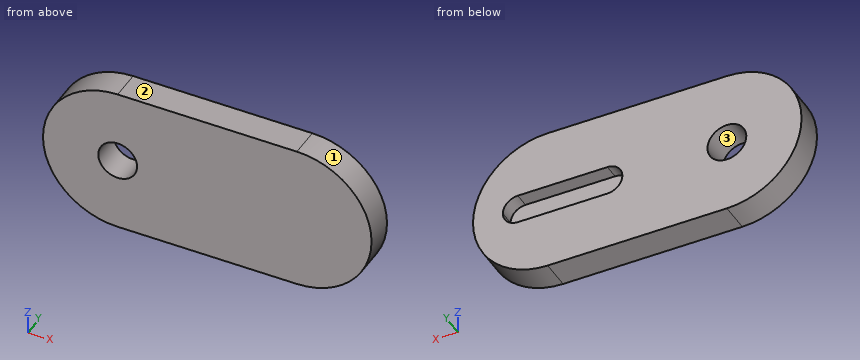
```python
from build123d import *

# Parameters (mm, degrees)
BOSS_EXTRUDE1_DEPTH = 2.54
SKETCH2_R           = 1.651
CUT_EXTRUDE1_DEPTH  = 2.54
SKETCH3_W           = 10.16
SKETCH3_H           = 2.54
CUT_EXTRUDE2_DEPTH  = 1.27
FILLET1_R           = 1.27


with BuildPart() as part:
    # Sketch1 → Boss-Extrude1 (new body)
    with BuildSketch(Plane(origin=(0, 0, 0), x_dir=(1, 0, 0), z_dir=(0, 1, 0))):
        with BuildLine():
            Line((0, 6.35), (15.24, 6.35))
            ThreePointArc((15.24, 6.35), (21.59, 0), (15.24, -6.35))
            Line((15.24, -6.35), (0, -6.35))
            ThreePointArc((0, -6.35), (-6.35, 0), (0, 6.35))
        make_face()
    extrude(amount=BOSS_EXTRUDE1_DEPTH)

    # Sketch2 → Cut-Extrude1 (cut)
    with BuildSketch(Plane(origin=(0, 2.54, 0), x_dir=(1, 0, 0), z_dir=(0, 1, 0))):
        with Locations(Location((0, 0, 0), (0, 0, 270))):
            Circle(SKETCH2_R)
    extrude(amount=-CUT_EXTRUDE1_DEPTH, mode=Mode.SUBTRACT)

    # Sketch3 → Cut-Extrude2 (cut)
    with BuildSketch(Plane(origin=(0, 2.54, 0), x_dir=(1, 0, 0), z_dir=(0, 1, 0))):
        with Locations((13.97, 0)):
            Rectangle(SKETCH3_W, SKETCH3_H)
    extrude(amount=-CUT_EXTRUDE2_DEPTH, mode=Mode.SUBTRACT)

    # Fillet1
    fillet1_edges = [part.edges().sort_by_distance(p)[0] for p in [
        (19.05, 1.905, 1.27),
        (19.05, 1.905, -1.27),
        (8.89, 1.905, 1.27),
        (8.89, 1.905, -1.27),
    ]]
    fillet(fillet1_edges, radius=FILLET1_R - 0.0001)  # a hair under: the kernel refuses the full size


solid = part.part
```
Check sheet for the modelled part. Datum: model origin and axes. Units: mm. Face numbers are marked on the shaded views. Give positions to 0.01 mm unless a question says otherwise; leave off trailing zeros. Loops run counter-clockwise (first coordinate to the right, second up) from the corner with the lowest first, then second, coordinate; pieces in that order, holes last. Notation, with made-up numbers: (-22.75, 9.5) - (34.25, 9.5) arc R16 cw to (34.25, 17.5) - close; hole circle Ø9 at (77, -38). An arc over 180 degrees is marked (long way). One line per question, with ' | ' between items. Start each with the question number.
1. Cross-section at B-B, the plane y = 1.55. Give the number of separate pieces and of enclosed holes in the cut face, plus the area to 3 significant figures.
2. Draft check along Z on the marked faces 1, 2 and 3. Enter one of: released by +Z, released by -Z, zero draft, split by the parting line, or undercut.
3. Material ranges on line 1 along X through (y, z) = (1.85, 0); line 2 along X through (y, z) = (1.2, 0); line 3 along Z through (x, y) = (11.75, 2.25), recorded low to high. Write a range as [from, to].
4. Gauge pin test, flat end, axial feed: pin 1 Ø4 at (x, z) = (13, -5) entering from -Y. Record the tip position at first contact, or that the pin passes through.
5. Cross-section at D-D, the plane z = 3. Enter the section's corners in (x, y), plus the area to 3 significant figures.
6. Cross-section at C-C, the plane x = -0.75. Enter the section's corners in (y, z), plus the area to 3 significant figures.
7. Cross-section at A-A, the plane x = 12.5. Enter the section's corners in (y, z).
Check result:
1) separate pieces: 1 | enclosed holes: 2 | area: 287 mm2
2) face 1: split by the parting line | face 2: released by +Z | face 3: undercut
3) line 1: x = [-6.35, -1.65], [1.65, 8.89], [19.05, 21.59] | line 2: x = [-6.35, -1.65], [1.65, 21.59] | line 3: z = [-6.35, -1.27], [1.27, 6.35]
4) pin 1: stops at y = 0
5) outline: (-5.6, 0) - (20.84, 0) - (20.84, 2.54) - (-5.6, 2.54) - close | area: 67.1 mm2
6) outline: (0, -6.31) - (2.54, -6.31) - (2.54, -1.47) - (0, -1.47) - close; (0, 1.47) - (2.54, 1.47) - (2.54, 6.31) - (0, 6.31) - close | area: 24.6 mm2
7) outline: (0, -6.35) - (2.54, -6.35) - (2.54, -1.27) - (1.27, -1.27) - (1.27, 1.27) - (2.54, 1.27) - (2.54, 6.35) - (0, 6.35) - close
